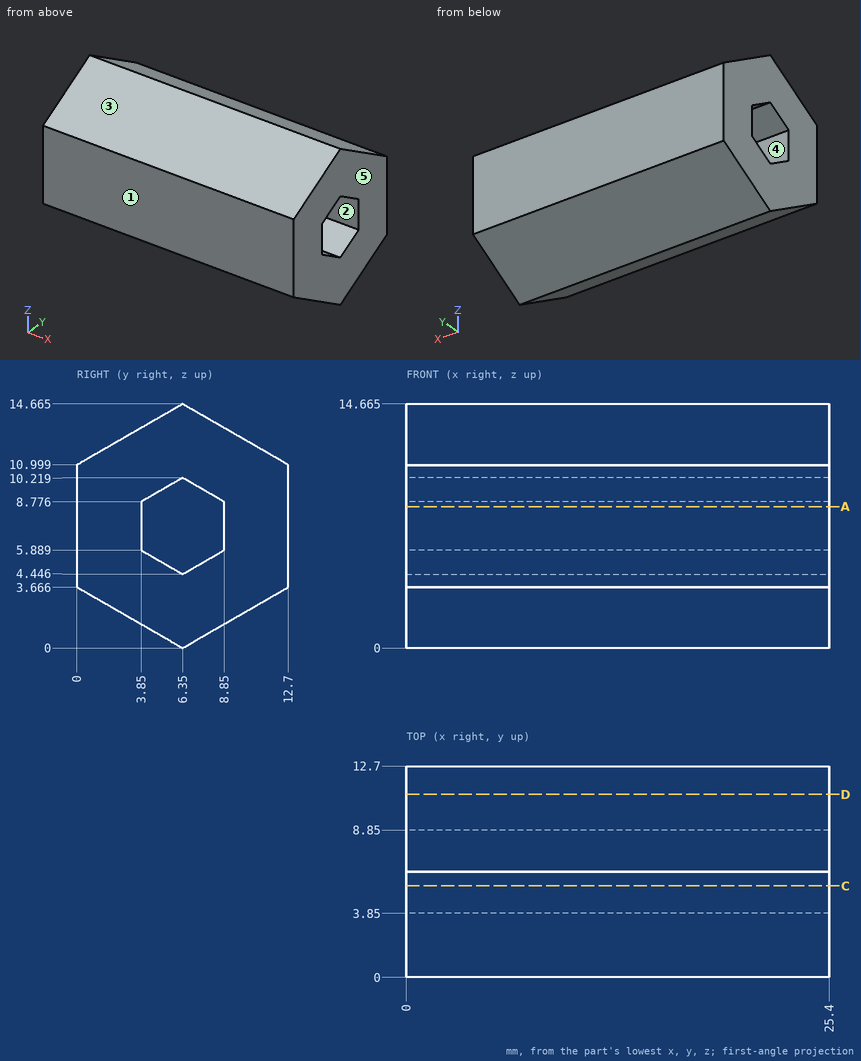
Check sheet for the drawn part. Datum: minimum x, y, z corner. Units: mm. A direction names the side the tool comes from. Round coordinates to 2 decimals unless told otherwise and drop trailing zeros. Order: outer loops, then holes, each group sorted by start corner. A loop starts at its lowest first (then second) coordinate and runs counter-clockwise, first axis right, second up. Notation, with made-up numbers: (84.25, -39.75) -> (91.25, -39.75) arc R32 ccw to (91.25, -4.75) -> close; hole circle Ø11 at (-21.5, 88.5). An arc over 180 degrees is marked (long way). Put each result on its own line as item: value.
1) Section check D-D (y = 11). Record the cut outline in (x, z) (1 decimal).
Final values:
outline: (0, 2.7) -> (25.4, 2.7) -> (25.4, 12) -> (0, 12) -> close
2) Depth check by flat-ended pin: pin 1 (4 mm diameter, centred on x = 22.5, z = 5.5, fed in from -Y); pin 2 (3 mm diameter, centred on x = 20, y = 8.5, fed in from -Z) (1 decimal); pin 3 (1 mm diameter, centred on x = 18.5, y = 5.5, fed in from -Z); pin 4 (2 mm diameter, centred on x = 22.5, y = 9, fed in from -Z). Enter the tip coordinate at first touch or a pass-through.
Final values:
pin 1: stops at y = 0
pin 2: stops at z = 0.4
pin 3: stops at z = 0.2
pin 4: stops at z = 0.95
3) Section check C-C (y = 5.5). Record the cut outline in (x, z).
Final values:
outline: (0, 0.49) -> (25.4, 0.49) -> (25.4, 4.94) -> (0, 4.94) -> close; (0, 9.73) -> (25.4, 9.73) -> (25.4, 14.17) -> (0, 14.17) -> close
4) Section check A-A (z = 8.5). Record the cut outline in (x, y).
Final values:
outline: (0, 0) -> (25.4, 0) -> (25.4, 3.85) -> (0, 3.85) -> close; (0, 8.85) -> (25.4, 8.85) -> (25.4, 12.7) -> (0, 12.7) -> close
5) Set-up check for the marked faces 1 and 2: record each of +Z, -Z, +X, -X, +Y, -Y from which the full face is reachable in a straight line by a thin tool's end or side.
Final values:
face 1: +Z, -Z, +X, -X, -Y
face 2: +X, -X
6) Material ranges on line 1 (Y direction, x = 13.5, z = 7); line 2 (Z direction, x = 12.5, y = 7.75) (1 decimal); line 3 (Z direction, x = 9, y = 5.5) (1 decimal), recorded low to high.
Final values:
line 1: y = 0 to 3.85, 8.85 to 12.7
line 2: z = 0.8 to 5.3, 9.4 to 13.9
line 3: z = 0.5 to 4.9, 9.7 to 14.2
7) Mould release check, pull along Y, two halves, no side actions. Record for the marked faces 3, 4 and 5: +Y half, -Y half, draft (parallel to the pull), parting line (faces both ways), or undercut.
Final values:
face 3: -Y half
face 4: undercut
face 5: draft
